Could you check a few things on this model? Use its own coordinates, in mm. A direction names the side the tool comes from. Coordinates: 2 decimals unless noted, no trailing zeros. Write each loop counter-clockwise with the first axis right and the second up, starting at its lowest first coordinate (ties: lowest second). Pieces come first, ordered by that corner, then holes.
```python
from build123d import *

# Parameters (mm, degrees)
SKETCH1_R           = 3
BOSS_EXTRUDE1_DEPTH = 120


with BuildPart() as part:
    # Sketch1 → Boss-Extrude1 (new body)
    with BuildSketch(Plane.XY):
        Circle(SKETCH1_R)
    extrude(amount=BOSS_EXTRUDE1_DEPTH)

    # Sketch3 → M4x0.7 Tapped Hole1 (revolve, cut)
    with BuildSketch(Plane(origin=(0, 0, 120), x_dir=(0, -1, 0), z_dir=(1, 0, 0))):
        Polygon((0, 0), (0, 10.991420021), (1.65, 10), (1.65, 0), align=None)
    m4x0_7_tapped_hole1 = revolve(axis=Axis((0, 0, 126.35), (0, 0, -1)), mode=Mode.SUBTRACT)

    # Mirror1: M4x0.7 Tapped Hole1 across plane
    add(m4x0_7_tapped_hole1.mirror(Plane.XY.offset(60)), mode=Mode.SUBTRACT)


solid = part.part
```
1. Please list where these lines run through material, in increasing order: line 1 along Y through (x, z) = (0, 6.25); line 2 along X through (y, z) = (-0.15, 52.5); line 3 along X through (y, z) = (-0.8, 61.5).
Verdict:
line 1: y = -3 to -1.65, 1.65 to 3
line 2: x = -3 to 3
line 3: x = -2.89 to 2.89
2. For pin 1 (2 mm diameter, centred on x = 0, y = 0, fed in from -Z); pin 2 (1.5 mm diameter, centred on x = -1.5, z = 107.5, fed in from +Y); pin 3 (1.5 mm diameter, centred on y = -2.5, z = 29.5, fed in from -X), each with a flat end and sliding along its axis, tell me the tip position at first contact or that it passes through.
Verdict:
pin 1: stops at z = 10.39
pin 2: stops at y = 2.9
pin 3: stops at x = -2.44
3. If we mould it in two halves opening along X, with no side actions, what happens to faces 1 (the face through (-3, 0, 59)), 2 (the face through (-1.115, 1.216, 4.93)), 3 (the face through (1.3, -1.3, 120))? For each: pulls with the +X half, pulls with the -X half, needs draft (parallel to the pull), parting line crosses it, or undercut.
Verdict:
face 1: parting line crosses it
face 2: undercut
face 3: needs draft
4. I want a section at A-A on z = 38. Please give me the cut outline in (x, y).
Verdict:
outline: circle Ø6 at (0, 0)
5. On a 3-axis mill with a long thin cutter (end or side, diameter ignored), from which of +Z, -Z, +X, -X, +Y, -Y can I reach the whole of each face in a straight line? I mean faces 4 (the face through (0.3, 0.1, 10.8)), 5 (the face through (-1.115, 1.216, 115.07)). Say none if no direction works.
Verdict:
face 4: -Z
face 5: +Z
